```python
from build123d import *

# Parameters (mm, degrees)
SKETCH1_W           = 164
SKETCH1_H           = 55
SKETCH1_W_2         = 15
SKETCH1_H_2         = 2.5
BOSS_EXTRUDE1_DEPTH = 3
CUT_EXTRUDE1_DEPTH  = 3
SKETCH3_R           = 1.25
CUT_EXTRUDE2_DEPTH  = 10
SKETCH4_R           = 2.5
CUT_EXTRUDE3_DEPTH  = 4
SKETCH5_R           = 1.63582752
SKETCH5_R_2         = 1.550817753
SKETCH5_R_3         = 1.410083192
SKETCH5_R_4         = 1.692495787
CUT_EXTRUDE4_DEPTH  = 4


with BuildPart() as part:
    # Sketch1 → Boss-Extrude1 (new body)
    with BuildSketch(Plane(origin=(0, 0, 0), x_dir=(1, 0, 0), z_dir=(0, 1, 0))):
        Rectangle(SKETCH1_W, SKETCH1_H)
        with Locations((48.5, 14.5)):
            Rectangle(SKETCH1_W_2, SKETCH1_H_2, mode=Mode.SUBTRACT)
        with Locations((68.5, 14.5)):
            Rectangle(SKETCH1_W_2, SKETCH1_H_2, mode=Mode.SUBTRACT)
        with Locations((68.5, -14.5)):
            Rectangle(SKETCH1_W_2, SKETCH1_H_2, mode=Mode.SUBTRACT)
        with Locations((48.5, -14.5)):
            Rectangle(SKETCH1_W_2, SKETCH1_H_2, mode=Mode.SUBTRACT)
        with Locations((-48.5, -14.5)):
            Rectangle(SKETCH1_W_2, SKETCH1_H_2, mode=Mode.SUBTRACT)
        with Locations((-68.5, -14.5)):
            Rectangle(SKETCH1_W_2, SKETCH1_H_2, mode=Mode.SUBTRACT)
        with Locations((-68.5, 14.5)):
            Rectangle(SKETCH1_W_2, SKETCH1_H_2, mode=Mode.SUBTRACT)
        with Locations((-48.5, 14.5)):
            Rectangle(SKETCH1_W_2, SKETCH1_H_2, mode=Mode.SUBTRACT)
    extrude(amount=BOSS_EXTRUDE1_DEPTH)

    # Sketch2 → Cut-Extrude1 (cut)
    with BuildSketch(Plane(origin=(0, 3, 0), x_dir=(1, 0, 0), z_dir=(0, 1, 0))):
        with BuildLine():
            Line((-31.658505885, 2), (-8.266387648, 2))
            ThreePointArc((-8.266387648, 2), (-6.266387648, 0), (-8.266387648, -2))
            Line((-8.266387648, -2), (-31.658505885, -2))
            ThreePointArc((-31.658505885, -2), (-33.658505885, 0), (-31.658505885, 2))
        make_face()
        with BuildLine():
            Line((31.658505885, -9.856733432), (8.266387648, -9.856733432))
            ThreePointArc((8.266387648, -9.856733432), (6.266387648, -7.856733432), (8.266387648, -5.856733432))
            Line((8.266387648, -5.856733432), (31.658505885, -5.856733432))
            ThreePointArc((31.658505885, -5.856733432), (33.658505885, -7.856733432), (31.658505885, -9.856733432))
        make_face()
        with BuildLine():
            Line((-31.658505885, 9.620758334), (-8.266387648, 9.620758334))
            ThreePointArc((-8.266387648, 9.620758334), (-6.266387648, 7.620758334), (-8.266387648, 5.620758334))
            Line((-8.266387648, 5.620758334), (-31.658505885, 5.620758334))
            ThreePointArc((-31.658505885, 5.620758334), (-33.658505885, 7.620758334), (-31.658505885, 9.620758334))
        make_face()
        with BuildLine():
            Line((31.658505885, 5.620758334), (8.266387648, 5.620758334))
            ThreePointArc((8.266387648, 5.620758334), (6.266387648, 7.620758334), (8.266387648, 9.620758334))
            Line((8.266387648, 9.620758334), (31.658505885, 9.620758334))
            ThreePointArc((31.658505885, 9.620758334), (33.658505885, 7.620758334), (31.658505885, 5.620758334))
        make_face()
        with BuildLine():
            Line((-31.658505885, -5.856733432), (-8.266387648, -5.856733432))
            ThreePointArc((-8.266387648, -5.856733432), (-6.266387648, -7.856733432), (-8.266387648, -9.856733432))
            Line((-8.266387648, -9.856733432), (-31.658505885, -9.856733432))
            ThreePointArc((-31.658505885, -9.856733432), (-33.658505885, -7.856733432), (-31.658505885, -5.856733432))
        make_face()
        with BuildLine():
            Line((31.658505885, -2), (8.266387648, -2))
            ThreePointArc((8.266387648, -2), (6.266387648, 0), (8.266387648, 2))
            Line((8.266387648, 2), (31.658505885, 2))
            ThreePointArc((31.658505885, 2), (33.658505885, 0), (31.658505885, -2))
        make_face()
    extrude(amount=-CUT_EXTRUDE1_DEPTH, mode=Mode.SUBTRACT)

    # Sketch3 → Cut-Extrude2 (cut)
    with BuildSketch(Plane(origin=(0, 3, 0), x_dir=(1, 0, 0), z_dir=(0, 1, 0))):
        with Locations((40, 18.5)):
            Circle(SKETCH3_R)
        with Locations((40, -18.5)):
            Circle(SKETCH3_R)
        with Locations((3, -18.5)):
            Circle(SKETCH3_R)
        with Locations((3, 18.5)):
            Circle(SKETCH3_R)
    extrude(amount=-CUT_EXTRUDE2_DEPTH, mode=Mode.SUBTRACT)

    # Sketch4 → Cut-Extrude3 (cut, through all)
    with BuildSketch(Plane(origin=(0, 3, 0), x_dir=(1, 0, 0), z_dir=(0, 1, 0))):
        with Locations((72, -22.5)):
            Circle(SKETCH4_R)
        with Locations((62, -22.5)):
            Circle(SKETCH4_R)
        with Locations((72, 22.5)):
            Circle(SKETCH4_R)
        with Locations((62, 22.5)):
            Circle(SKETCH4_R)
        with Locations((-72, 22.5)):
            Circle(SKETCH4_R)
        with Locations((-62, 22.5)):
            Circle(SKETCH4_R)
        with Locations((-72, -22.5)):
            Circle(SKETCH4_R)
        with Locations((-62, -22.5)):
            Circle(SKETCH4_R)
    extrude(amount=-CUT_EXTRUDE3_DEPTH, mode=Mode.SUBTRACT)

    # Sketch5 → Cut-Extrude4 (cut, through all)
    with BuildSketch(Plane(origin=(0, 3, 0), x_dir=(1, 0, 0), z_dir=(0, 1, 0))):
        with Locations((34.323103301, -23.81549711)):
            Circle(SKETCH5_R)
        with Locations((35.235754497, 23.565498985)):
            Circle(SKETCH5_R_2)
        with Locations((-45.484369153, 23.437784188)):
            Circle(SKETCH5_R_3)
        with Locations((-39.276258797, -23.81549711)):
            Circle(SKETCH5_R_4)
    extrude(amount=-CUT_EXTRUDE4_DEPTH, mode=Mode.SUBTRACT)


solid = part.part
```
Design review of the part built by this model. Coordinates are the model's own, in mm. A direction names the side the tool comes from. Give positions to 0.01 mm unless a question says otherwise; leave off trailing zeros. Order: outer loops, then holes, each group sorted by start corner. A loop starts at its lowest first (then second) coordinate and runs counter-clockwise, first axis right, second up. Notation, with made-up numbers: (62, 83.25) -> (100, 83.25) arc R19 ccw to (100, 99.25) -> close; hole circle Ø1 at (5.5, -19). An arc over 180 degrees is marked (long way). Write item = value, one per line. Start each with the question number.
(1) We need section D-D on x = 72.5. Write out the cut boundary in (y, z), plus the area to 3 significant figures.
(2) Mouldability with a two-part tool opening along X and no side actions: class faces 1 (the face through (20, 2, -5.621)), 2 (the face through (-1, 1, -27.5)) as +X half, -X half, draft (parallel to the pull), parting line (faces both ways), or undercut.
(3) We need section B-B on z = 0. Write out the cut boundary in (x, y).
(4) We need section C-C on x = 25. Write out the cut boundary in (y, z), plus the area to 3 significant figures.
(5) To check wall thickness, follow line 1 along X through (y, z) = (2.35, -18.5); line 2 along Z through (x, y) = (40, 0.75); line 3 along X through (y, z) = (1.75, 15.5). State the ranges of each line that lie inside material, in increasing order.
(6) For faces 3 (the face through (-20, 2, -9.621)), 4 (the face through (-1, 0, 0)), list the 3-axis set-ups (+Z, -Z, +X, -X, +Y, -Y) from which the entire face can be reached by the end or side of a thin tool; tool diameter is ignored.
(7) We need section A-A on x = -72. Write out the cut boundary in (y, z).
Numbers:
q1.outline = (0, -27.5) -> (3, -27.5) -> (3, -24.95) -> (0, -24.95) -> close; (0, -20.05) -> (3, -20.05) -> (3, -15.75) -> (0, -15.75) -> close; (0, -13.25) -> (3, -13.25) -> (3, 13.25) -> (0, 13.25) -> close; (0, 15.75) -> (3, 15.75) -> (3, 20.05) -> (0, 20.05) -> close; (0, 24.95) -> (3, 24.95) -> (3, 27.5) -> (0, 27.5) -> close
q1.area = 121 mm^2
q2.face_1 = undercut
q2.face_2 = draft
q3.outline = (-82, 0) -> (-33.66, 0) -> (-33.66, 3) -> (-82, 3) -> close; (-6.27, 0) -> (6.27, 0) -> (6.27, 3) -> (-6.27, 3) -> close; (33.66, 0) -> (82, 0) -> (82, 3) -> (33.66, 3) -> close
q4.outline = (0, -27.5) -> (3, -27.5) -> (3, -9.62) -> (0, -9.62) -> close; (0, -5.62) -> (3, -5.62) -> (3, -2) -> (0, -2) -> close; (0, 2) -> (3, 2) -> (3, 5.86) -> (0, 5.86) -> close; (0, 9.86) -> (3, 9.86) -> (3, 27.5) -> (0, 27.5) -> close
q4.area = 129 mm^2
q5.line_1 = -82 to 1.75, 4.25 to 38.75, 41.25 to 82
q5.line_2 = -27.5 to -19.75, -17.25 to 17.25, 19.75 to 27.5
q5.line_3 = -82 to -76, -61 to -56, -41 to 41, 56 to 61, 76 to 82
q6.face_3 = +Y, -Y
q6.face_4 = +Z, -Z, +X, -X, -Y
q7.outline = (0, -27.5) -> (3, -27.5) -> (3, -25) -> (0, -25) -> close; (0, -20) -> (3, -20) -> (3, -15.75) -> (0, -15.75) -> close; (0, -13.25) -> (3, -13.25) -> (3, 13.25) -> (0, 13.25) -> close; (0, 15.75) -> (3, 15.75) -> (3, 20) -> (0, 20) -> close; (0, 25) -> (3, 25) -> (3, 27.5) -> (0, 27.5) -> close
